The model under review builds one solid part; all positions refer to its coordinate system, in mm. Face numbers are marked on the shaded views. A direction names the side the tool comes from. Coordinates: 2 decimals unless noted, no trailing zeros. Loops run counter-clockwise (first coordinate to the right, second up) from the corner with the lowest first, then second, coordinate; pieces in that order, holes last. Notation, with made-up numbers: (58, 39) - (100, 39) arc R16 ccw to (100, 61) - close; hole circle Ø6 at (36, 68). An arc over 180 degrees is marked (long way). Answer in a Markdown table with one row per item. Add a question column.
(1) We need section C-C on x = 15. Write out the cut boundary in (y, z), plus the area to 3 significant figures.
(2) For P1, Ø0.7, axis at y = 42.5, z = 9, coming from the -X side; P2, Ø1, axis at y = 21, z = 4, coming from the -X side; P3, Ø1.8, axis at x = 33.5, z = 9, coming from the -Y side, all flat-tipped, find the tip position at first contact; note any pin that passes through.
(3) Mouldability with a two-part tool opening along X and no side actions: class the marked faces 5, 6, 7 and 8 as +X half, -X half, draft (parallel to the pull), parting line (faces both ways), or undercut.
(4) We need section D-D on y = 15. Write out the cut boundary in (x, z).
(5) We need section B-B on z = 3.75. Write out the cut boundary in (x, y), plus the area to 3 significant figures.
(6) Machinability: for the marked faces 1, 2, 3 and 4, which of the approach directions +Z, -Z, +X, -X, +Y, -Y give a long, thin tool a straight path to every point of the face, cutting with its end or side? Answer none if there is none.
(7) We need section A-A on y = 35.5. Write out the cut boundary in (x, z).
(8) For line 1 along Y through (x, z) = (27, 9.5); line 2 along Y through (x, z) = (14, 7); line 3 along Z through (x, y) = (17.5, 12), list the stretches that pass through material, from the lowest coordinate up.
from build123d import *

# Parameters (mm, degrees)
F0_W      = 60
F0_H      = 53.5
F1_DEPTH  = 2
F3_DEPTH  = 23.2
F4_W      = 15.2
F4_H      = 4
F5_DEPTH  = 2.2
F6_R      = 0.5
F8_DEPTH  = 20
F11_DEPTH = 2


with BuildPart() as f1:
    # F0 (on Top) → F1 (new body)
    with BuildSketch(Plane.XY):
        with Locations((30, 26.75)):
            Rectangle(F0_W, F0_H)
    extrude(amount=F1_DEPTH)

    # F2 (on face) → F3 (join)
    with BuildSketch(Plane(origin=(0, 53.5, 0), x_dir=(-1, 0, 0), z_dir=(0, 1, 0))):
        Polygon((-1.9529488989, 2), (-14, 8), (-46, 8), (-58.0470511011, 2), align=None)
    extrude(amount=-F3_DEPTH)

    # F4 (on face) → F5 (join)
    with BuildSketch(Plane.XY.offset(8)):
        with Locations((30, 48.9)):
            Rectangle(F4_W, F4_H)
        with Locations((30, 41.9)):
            Rectangle(F4_W, F4_H)
        with Locations((30, 34.9)):
            Rectangle(F4_W, F4_H)
    extrude(amount=F5_DEPTH)

    # F6
    f6_edges = [f1.edges().sort_by_distance(p)[0] for p in [
        (22.4, 46.9, 9.1),
        (22.4, 39.9, 9.1),
        (22.4, 32.9, 9.1),
        (22.4, 36.9, 9.1),
        (22.4, 43.9, 9.1),
        (22.4, 50.9, 9.1),
        (37.6, 32.9, 9.1),
        (37.6, 36.9, 9.1),
        (37.6, 39.9, 9.1),
        (37.6, 43.9, 9.1),
        (37.6, 46.9, 9.1),
        (37.6, 50.9, 9.1),
    ]]
    fillet(f6_edges, radius=F6_R)

    # F7 (on face) → F8 (join)
    with BuildSketch(Plane.XZ):
        Polygon((5, 2), (10, 2), (12.0235255505, 5), (11.0235255505, 5), align=None)
        Polygon((47.9764744495, 5), (50, 2), (55, 2), (48.9764744495, 5), align=None)
    extrude(amount=-F8_DEPTH)

    # F9 (on face) + F10 (on face) → F11 (join)
    with BuildSketch(Plane(origin=(0, 20, 0), x_dir=(-1, 0, 0), z_dir=(0, 1, 0))):
        Polygon((-10, 2), (-5, 2), (-11.0235255505, 5), (-12.0235255505, 5), align=None)
        Polygon((-12.0235255505, 2), (-10, 2), (-12.0235255505, 5), align=None)
    with BuildSketch(Plane(origin=(0, 20, 0), x_dir=(-1, 0, 0), z_dir=(0, 1, 0))):
        Polygon((-47.9764744495, 5), (-50, 2), (-47.9764744495, 2), align=None)
        Polygon((-48.9764744495, 5), (-55, 2), (-50, 2), (-47.9764744495, 5), align=None)
    extrude(amount=F11_DEPTH)


solid = f1.part
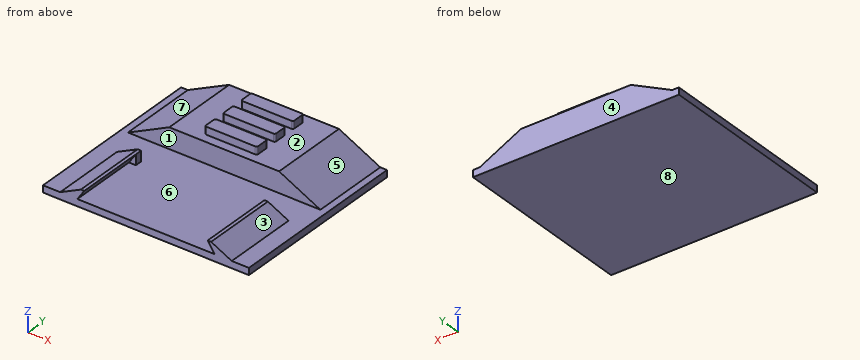
Outcome:
| question | item | result |
|---|---|---|
| 1 | outline | (0, 0) - (53.5, 0) - (53.5, 8) - (30.3, 8) - (30.3, 2) - (0, 2) - close |
| 1 | area | 246 mm² |
| 2 | P1 | x = 22.4 |
| 2 | P2 | x = 8.01 |
| 2 | P3 | y = 32.9 |
| 3 | face 5 | +X half |
| 3 | face 6 | undercut |
| 3 | face 7 | -X half |
| 3 | face 8 | draft |
| 4 | outline | (0, 0) - (60, 0) - (60, 2) - (55, 2) - (48.98, 5) - (47.98, 5) - (50, 2) - (10, 2) - (12.02, 5) - (11.02, 5) - (5, 2) - (0, 2) - close |
| 5 | outline | (5.47, 30.3) - (54.53, 30.3) - (54.53, 53.5) - (5.47, 53.5) - close; (8.51, 0) - (11.18, 0) - (11.18, 20) - (12.02, 20) - (12.02, 22) - (8.51, 22) - close; (47.98, 20) - (48.82, 20) - (48.82, 0) - (51.49, 0) - (51.49, 22) - (47.98, 22) - close |
| 5 | area | 1,260 mm² |
| 6 | face 1 | +Z, +X, -X |
| 6 | face 2 | +Z |
| 6 | face 3 | +Z, +X, -Y |
| 6 | face 4 | +Z, -Z, +X, -X, +Y |
| 7 | outline | (0, 0) - (60, 0) - (60, 2) - (58.05, 2) - (46, 8) - (37.6, 8) - (37.6, 10.2) - (22.4, 10.2) - (22.4, 8) - (14, 8) - (1.95, 2) - (0, 2) - close |
| 8 | line 1 | 32.9 to 36.9, 39.9 to 43.9, 46.9 to 50.9 |
| 8 | line 2 | 30.3 to 53.5 |
| 8 | line 3 | 0 to 2 |
